Input: part model. Units: mm. Frame: model coordinates. A direction names the side the tool comes from. Give positions to 0.01 mm unless a question says otherwise; leave off trailing zeros. Order: outer loops, then holes, each group sorted by start corner. A loop starts at its lowest first (then second) coordinate and runs counter-clockwise, first axis right, second up. Notation, with made-up numbers: (55, -23) - (78, -23) arc R24 cw to (78, -13) - close; hole circle Ø8 at (45, 67.5). An arc over 180 degrees is marked (long way). Answer in a Markdown table with one row per item. Add a question column.
from build123d import *

# Parameters (mm, degrees)
F0_R     = 32.5
F1_DEPTH = 10
F2_R     = 2.5
F3_T     = -1.5
F4_R     = 32.5
F4_R_2   = 31.75
F5_DEPTH = 2.5


# Not quite as in the source:
# - a feature names something its author has since deleted; it is built from what else it names


with BuildPart() as f1:
    # F0 (on Top) → F1 (new body)
    with BuildSketch(Plane.XY):
        Circle(F0_R)
    extrude(amount=F1_DEPTH)

    # F2
    f2_edges = [f1.edges().sort_by_distance(p)[0] for p in [
        (-32.5, 0, 0),
    ]]
    fillet(f2_edges, radius=F2_R)

    # F3
    f3_openings = [f1.faces().sort_by_distance(p)[0] for p in [
        (0, 0, 10),
    ]]
    offset(amount=F3_T, openings=f3_openings)

    # F4 (on face) → F5 (join)
    with BuildSketch(Plane.XY.offset(10)):
        Circle(F4_R)
        Circle(F4_R_2, mode=Mode.SUBTRACT)
    extrude(amount=F5_DEPTH)


solid = f1.part
Q1. Access query for faces 1 (the flat face through (7.1, -31.1, 12.5)), 2 (the flat face through (6.9, -30.4, 10)). Directions: +Z, -Z, +X, -X, +Y, -Y. A direction counts if a zero-diameter tool reaches every point of the face in a straight line with its end or side. Return the directions, or none.
Q2. Section C-C, the plane z = 3.25. Return loops of the section in (x, y), then the cut area to 3 significant figures.
Q3. Line query: probe 1 along Y at (x, z) = (0, 10.95); probe 2 along Y at (x, z) = (0, 5.25); probe 3 along Z at (x, y) = (-17.5, 22). Output: solid intervals per line, ascending.
Q4. Section A-A, the plane y = 0. Return loops of the section in (x, z), then the cut area to 3 significant figures.
Q5. Pull-direction query (X, two-part tool) for faces 3 (the cylindrical face through (31, 9.76, 7.43)), 4 (the cylindrical face through (-4.036, 30.736, 6.198)), 5 (the flat face through (0, 0, 0)); classes: +X half, -X half, draft (parallel to the pull), parting line (faces both ways), or undercut.
Q6. Contact query for flat-ended pins moving along their axis: P1, Ø6, axis at x = -14, z = 5, coming from the +Y side; P2, Ø6, axis at x = 25.5, z = 4.5, coming from the -Y side; P3, Ø18, axis at x = 4, y = 4.5, coming from the +Z side. Output: stop coordinate, or through.
Computed:
| question | item | result |
|---|---|---|
| 1 | face 1 | +Z, +X, -X, +Y, -Y |
| 1 | face 2 | +Z |
| 2 | outline | circle Ø65 at (0, 0); hole circle Ø62 at (0, 0) |
| 2 | area | 299 mm^2 |
| 3 | probe 1 | y = -32.5 to -31.75, 31.75 to 32.5 |
| 3 | probe 2 | y = -32.5 to -31, 31 to 32.5 |
| 3 | probe 3 | z = 0 to 1.5 |
| 4 | outline | (-32.5, 2.5) arc R2.5 ccw to (-30, 0) - (30, 0) arc R2.5 ccw to (32.5, 2.5) - (32.5, 12.5) - (31.75, 12.5) - (31.75, 10) - (31, 10) - (31, 2.5) arc R1 cw to (30, 1.5) - (-30, 1.5) arc R1 cw to (-31, 2.5) - (-31, 10) - (-31.75, 10) - (-31.75, 12.5) - (-32.5, 12.5) - close |
| 4 | area | 124 mm^2 |
| 5 | face 3 | parting line |
| 5 | face 4 | undercut |
| 5 | face 5 | draft |
| 6 | P1 | stops at y = 30.58 |
| 6 | P2 | stops at y = -23.45 |
| 6 | P3 | stops at z = 1.5 |
